```python
from build123d import *

# Parameters (mm, degrees)
SKETCH1_R           = 15.24
BOSS_EXTRUDE1_DEPTH = 6.35
SKETCH2_R           = 7.9375
CUT_EXTRUDE1_DEPTH  = 3.175
FILLET4_R           = 1.27
SKETCH4_R           = 1.5875
CUT_EXTRUDE2_DEPTH  = 2.54
CIRPATTERN1_COUNT   = 3
FILLET6_R           = 1.27
SKETCH3_R           = 3.0734
BOSS_EXTRUDE4_DEPTH = 11.43
FILLET7_R           = 1.27


with BuildPart() as part:
    # Sketch1 → Boss-Extrude1 (new body)
    with BuildSketch(Plane(origin=(0, 0, 0), x_dir=(1, 0, 0), z_dir=(0, 1, 0))):
        with Locations(Location((0, 0, 0), (0, 0, 270))):
            Circle(SKETCH1_R)
    extrude(amount=BOSS_EXTRUDE1_DEPTH)

    # Sketch2 → Cut-Extrude1 (cut)
    with BuildSketch(Plane(origin=(0, 6.35, 0), x_dir=(1, 0, 0), z_dir=(0, 1, 0))):
        with Locations(Location((0, 0, 0), (0, 0, 270))):
            Circle(SKETCH2_R)
    extrude(amount=-CUT_EXTRUDE1_DEPTH, mode=Mode.SUBTRACT)

    # Fillet4
    fillet4_edges = [part.edges().sort_by_distance(p)[0] for p in [
        (0, 6.35, -15.24),
    ]]
    fillet(fillet4_edges, radius=FILLET4_R)

    # Sketch4 → Cut-Extrude2 (cut)
    with BuildSketch(Plane(origin=(0, 6.35, 0), x_dir=(1, 0, 0), z_dir=(0, 1, 0))):
        with Locations(Location((0, 11.938, 0), (0, 0, 270))):
            Circle(SKETCH4_R)
    cut_extrude2 = extrude(amount=-CUT_EXTRUDE2_DEPTH, mode=Mode.SUBTRACT)

    # CirPattern1: Cut-Extrude2 ×3 about axis
    cirpattern1_axis = Axis((0, 0, 0), (0, 1, 0))
    for i in range(1, CIRPATTERN1_COUNT):
        add(cut_extrude2.rotate(cirpattern1_axis, i * 360 / CIRPATTERN1_COUNT), mode=Mode.SUBTRACT)

    # Fillet6
    fillet6_edges = [part.edges().sort_by_distance(p)[0] for p in [
        (0, 0, -15.24),
    ]]
    fillet(fillet6_edges, radius=FILLET6_R)

    # Sketch3 → Boss-Extrude4 (add)
    with BuildSketch(Plane.XZ):
        with Locations(Location((0, 0, 0), (0, 0, 90))):
            Circle(SKETCH3_R)
    extrude(amount=BOSS_EXTRUDE4_DEPTH)

    # Fillet7
    fillet7_edges = [part.edges().sort_by_distance(p)[0] for p in [
        (0, 0, -3.0734),
        (0, -11.43, -3.0734),
    ]]
    fillet(fillet7_edges, radius=FILLET7_R)


solid = part.part
```
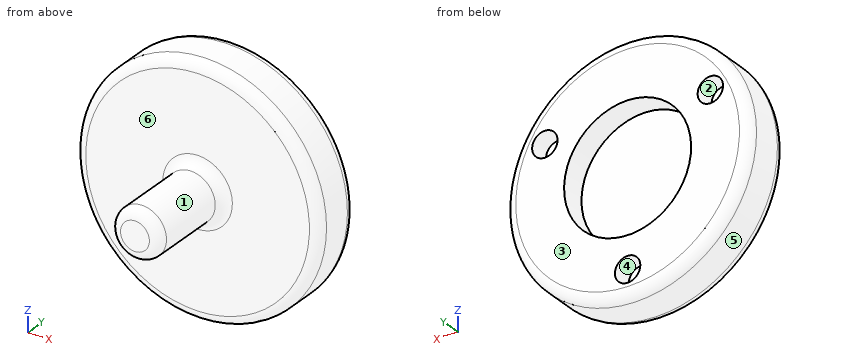
The listing builds one solid part. Answer for the finished solid, in the listing's coordinates (mm). Face numbers are marked on the shaded views. A direction names the side the tool comes from. Coordinates: 2 decimals unless noted, no trailing zeros. Write each loop counter-clockwise with the first axis right and the second up, starting at its lowest first coordinate (ties: lowest second). Pieces come first, ordered by that corner, then holes. Notation, with made-up numbers: (-6, 46) - (14, 46) arc R27 cw to (14, 84) - close; hole circle Ø8 at (-37, 20.25). An arc over 180 degrees is marked (long way). Return JSON: item names as keys, results as strings. Group by question number.
Q1. Which of the six approach directions +Z, -Z, +X, -X, +Y, -Y give full straight-line access (tool end or side, diameter ignored) to the marked faces 4, 5 and 6?
Q2. For a pull along Z with two mould halves and no side action, classify the marked faces 1, 2 and 3 as +Z half, -Z half, draft (parallel to the pull), parting line (faces both ways), or undercut.
Q3. Flat-ended cylindrical pins translate along their axes: pin 1 Ø1.6 at (x, z) = (-10, 5.5) entering from +Y; pin 2 Ø5 at (x, y) = (11.5, -4) entering from -Z; pin 3 Ø4 at (x, z) = (0, -11.938) entering from -Y; pin 4 Ø8.5 at (x, z) = (5, 2) entering from -Y. Find the tip coordinate at first contact, or state that the pin passes through.
Q4. The part is cut by section C-C on y = 2.5. Write down the section's boundary in (x, z).
Q5. The part is cut by section D-D on y = -4.5. Write down the section's boundary in (x, z), and give its area (3 significant figures).
Q6. Find the intervals of material crossed by line 1 along X through (y, z) = (5.25, 6); line 2 along X through (y, z) = (4, 0); line 3 along Y through (x, z) = (11.5, 1), in increasing order. Write a range as [from, to].
Evaluation:
{
 "1": {"face 4": "+Y", "face 5": "+Y, -Y", "face 6": "-Y"},
 "2": {"face 1": "parting line", "face 2": "undercut", "face 3": "draft"},
 "3": {"pin 1": "stops at y = 3.81", "pin 2": "passes through", "pin 3": "stops at y = 0", "pin 4": "stops at y = -11.43"},
 "4": {"outline": "circle Ø30.48 at (0, 0)"},
 "5": {"outline": "circle Ø6.15 at (0, 0)", "area": "29.7 mm2"},
 "6": {"line 1": "x = [-14, -11.93], [-8.75, -5.2], [5.2, 8.75], [11.93, 14]", "line 2": "x = [-15.24, -7.94], [7.94, 15.24]", "line 3": "y = [0, 6.35]"}
}
